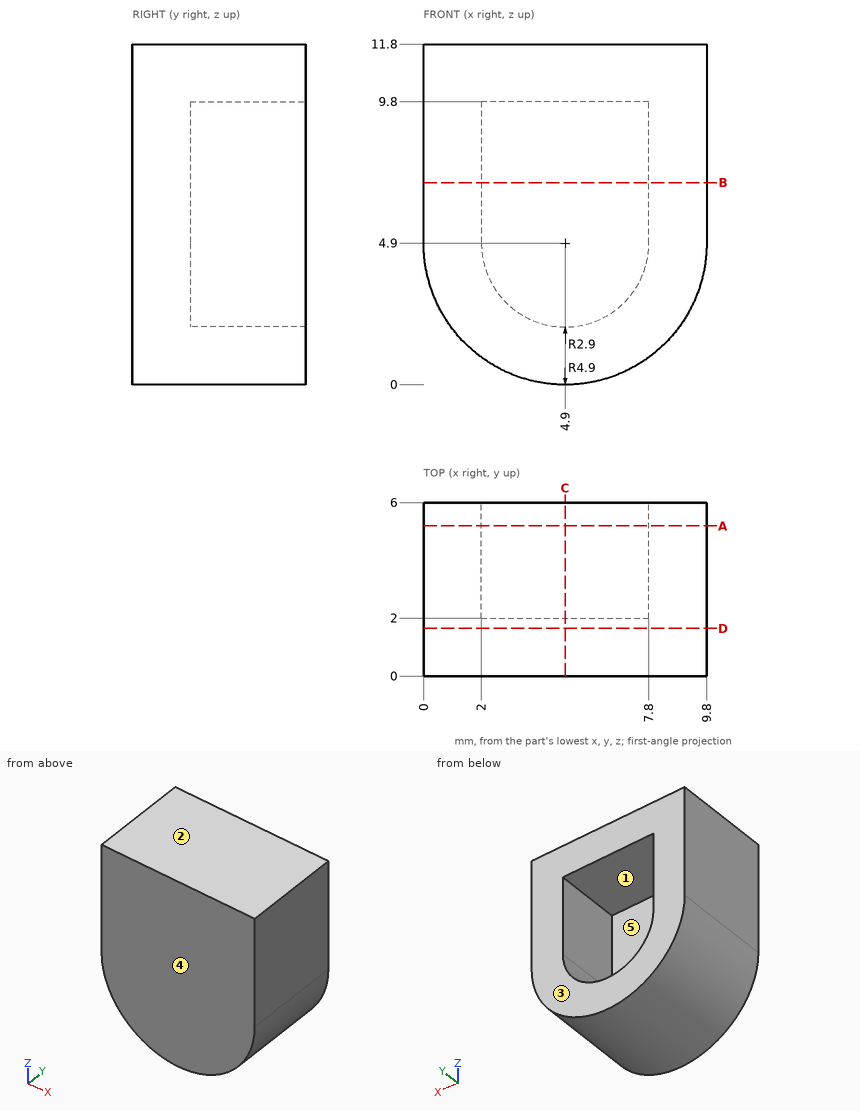
Source: three-view drawing plus pictorial views. Frame: mm from the lowest corner of the part. A direction names the side the tool comes from. Give positions to 0.01 mm unless a question says otherwise; leave off trailing zeros. Order: outer loops, then holes, each group sorted by start corner. A loop starts at its lowest first (then second) coordinate and runs counter-clockwise, first axis right, second up. Notation, with made-up numbers: M 1,-10 L 17,-10 A21 ccw 17,13 Z; hole C 51.25,28 d11. An arc over 180 degrees is marked long. One line per question, with ' | ' between items. Start each with the question number.
1. Section query D-D (y = 1.65). Return the cut outline in (x, z), and give its area (3 significant figures).
2. Section query A-A (y = 5.2). Return the cut outline in (x, z).
3. Section query B-B (z = 7). Return the cut outline in (x, y), and give its area (3 significant figures).
4. Pull-direction query (Z, two-part tool) for the marked faces 1, 2 and 3; classes: released by +Z, released by -Z, zero draft, split by the parting line, or undercut.
5. Access query for the marked faces 4 and 5. Directions: +Z, -Z, +X, -X, +Y, -Y. A direction counts if a zero-diameter tool reaches every point of the face in a straight line with its end or side. Return the directions, or none.
6. Section query C-C (x = 4.9). Return the cut outline in (y, z).
7. Material intervals for probe 1 along X at (y, z) = (2.85, 6.75); probe 2 along Z at (x, y) = (5, 3); probe 3 along Z at (x, y) = (7.5, 5.25), sorted ascending. Write a range as [from, to].
8. First-contact query: pin 1 Ø3 at (x, z) = (5.5, 6) entering from +Y. Flat tip, straight axial feed; report the tip coordinate or a pass-through.
Here are the results:
1) outline: M 0,4.9 A4.9 ccw 9.8,4.9 L 9.8,11.8 L 0,11.8 Z | area: 105 mm²
2) outline: M 0,4.9 A4.9 ccw 9.8,4.9 L 9.8,11.8 L 0,11.8 Z; hole M 2,4.9 A2.9 ccw 7.8,4.9 L 7.8,9.8 L 2,9.8 Z
3) outline: M 0,0 L 9.8,0 L 9.8,6 L 7.8,6 L 7.8,2 L 2,2 L 2,6 L 0,6 Z | area: 35.6 mm²
4) face 1: undercut | face 2: released by +Z | face 3: zero draft
5) face 4: +Z, -Z, +X, -X, -Y | face 5: +Y
6) outline: M 0,0 L 6,0 L 6,2 L 2,2 L 2,9.8 L 6,9.8 L 6,11.8 L 0,11.8 Z
7) probe 1: [0, 2], [7.8, 9.8] | probe 2: [0, 2], [9.8, 11.8] | probe 3: [0.75, 3.62], [9.8, 11.8]
8) pin 1: y = 2
